Check sheet for the modelled part. Datum: model origin and axes. Units: mm. A direction names the side the tool comes from. Coordinates: 2 decimals unless noted, no trailing zeros. Order: outer loops, then holes, each group sorted by start corner. A loop starts at its lowest first (then second) coordinate and runs counter-clockwise, first axis right, second up.
1. Cross-section at D-D (x = -5.25). Enter the section's corners in (y, z), then the cut area to 3 significant figures.
2. Thickness scan on line 1 (Z direction, x = 5.25, y = 4); line 2 (X direction, y = 5, z = 4.5); line 3 (Y direction, x = -4, z = 6.5). Record the ranges inside material, lowest first.
3. Set-up check for faces 1 (the flat face through (0, 0, 10)), 2 (the cylindrical face through (-1.08, -4.88, 3.94)): record each of +Z, -Z, +X, -X, +Y, -Y from which the full face is reachable in a straight line by a thin tool's end or side.
4. Cross-section at A-A (y = 0). Enter the section's corners in (x, z).
5. Cross-section at C-C (z = -1.75). Enter the section's corners in (x, y), then the cut area to 3 significant figures.
6. Gauge pin test, flat ends, axial feed: pin 1 Ø4 at (y, z) = (-2.5, -3) entering from +X; pin 2 Ø3 at (y, z) = (3, 4.5) entering from +X; pin 3 Ø3 at (x, z) = (-3, 4.5) entering from -Y. Record the tip position at first contact, or that the pin passes through.
7. Cross-section at B-B (x = 0). Enter the section's corners in (y, z).
```python
from build123d import *

# Parameters (mm, degrees)
SKETCH_1_R      = 5
EXTRUDE_1_DEPTH = 10
SKETCH_2_R      = 7.5
EXTRUDE_2_DEPTH = 5
FILLET_1_R      = 2
SKETCH_5_R      = 1.5
EXTRUDE_4_DEPTH = 5


with BuildPart() as part:
    # 草图1 → 凸台-拉伸1 (new body)
    with BuildSketch(Plane.XY):
        Circle(SKETCH_1_R)
    extrude(amount=EXTRUDE_1_DEPTH)

    # 草图2 → 凸台-拉伸2 (add)
    with BuildSketch(Plane(origin=(0, 0, 0), x_dir=(-1, 0, 0), z_dir=(0, 0, -1))):
        Circle(SKETCH_2_R)
    extrude(amount=EXTRUDE_2_DEPTH)

    # 圆角1
    fillet_1_edges = [part.edges().sort_by_distance(p)[0] for p in [
        (-5, 0, 10),
    ]]
    fillet(fillet_1_edges, radius=FILLET_1_R)

    # 草图5 → 凸台-拉伸4 (add)
    with BuildSketch(Plane.XY):
        with Locations((0, 5)):
            Circle(SKETCH_5_R)
    extrude(amount=EXTRUDE_4_DEPTH)


solid = part.part
```
Data:
1. outline: (-5.36, -5) - (5.36, -5) - (5.36, 0) - (-5.36, 0) - close
1. area: 53.6 mm2
2. line 1: z = -5 to 0
2. line 2: x = -1.5 to 1.5
2. line 3: y = -3 to 3
3. face 1: +Z, +X, -X, +Y, -Y
3. face 2: +Z
4. outline: (-7.5, -5) - (7.5, -5) - (7.5, 0) - (5, 0) - (5, 8) arc R2 ccw to (3, 10) - (-3, 10) arc R2 ccw to (-5, 8) - (-5, 0) - (-7.5, 0) - close
5. outline: circle Ø15 at (0, 0)
5. area: 177 mm2
6. pin 1: stops at x = 7.48
6. pin 2: stops at x = 4.77
6. pin 3: stops at y = -4.77
7. outline: (-7.5, -5) - (7.5, -5) - (7.5, 0) - (6.5, 0) - (6.5, 5) - (5, 5) - (5, 8) arc R2 ccw to (3, 10) - (-3, 10) arc R2 ccw to (-5, 8) - (-5, 0) - (-7.5, 0) - close
